Check sheet for the modelled part. Datum: model origin and axes. Units: mm. Coordinates: 2 decimals unless noted, no trailing zeros. Order: outer loops, then holes, each group sorted by start corner. A loop starts at its lowest first (then second) coordinate and runs counter-clockwise, first axis right, second up.
from build123d import *

# Parameters (mm, degrees)
SM_BASE_FLANGE_1_DEPTH      = 746
HOLE_WIZARD_M41_D           = 3.3
HOLE_WIZARD_M41_DEPTH       = 11.5
HOLE_WIZARD_M41_CSINK_D     = 4.05
HOLE_WIZARD_M41_CSINK_ANGLE = 90
HOLE_WIZARD_M41_TIP         = 0.991420021
HOLE_WIZARD_M61_D           = 6.6
HOLE_WIZARD_M61_DEPTH       = 59
HOLE_WIZARD_M61_TIP         = 1.982840043


# Sheet-metal steps are written as plain solids
with BuildPart() as part:
    # Sketch 1 → Базовая кромка1 (new body)
    with BuildSketch(Plane.XY):
        with BuildLine():
            Line((0, 40), (0, 3.8))
            ThreePointArc((0, 3.8), (1.112994231, 1.112994231), (3.8, 0))
            Line((3.8, 0), (30, 0))
            Line((30, 0), (30, 2))
            Line((30, 2), (3.8, 2))
            ThreePointArc((3.8, 2), (2.527207794, 2.527207794), (2, 3.8))
            Line((2, 3.8), (2, 40))
            Line((2, 40), (0, 40))
        make_face()
    extrude(amount=SM_BASE_FLANGE_1_DEPTH)

    # Отверстие обработанное метчиком M41
    with Locations(Plane(origin=(0, 0, 0), x_dir=(-1, 0, 0), z_dir=(0, -1, 0))):
        with Locations((-15, -18), (-15, -89), (-15, -160), (-15, -231), (-15, -302), (-15, -373), (-15, -444), (-15, -515), (-15, -586), (-15, -657), (-15, -728)):
            CounterSinkHole(HOLE_WIZARD_M41_D / 2, HOLE_WIZARD_M41_CSINK_D / 2, depth=HOLE_WIZARD_M41_DEPTH, counter_sink_angle=HOLE_WIZARD_M41_CSINK_ANGLE)
            with Locations((0, 0, -(HOLE_WIZARD_M41_DEPTH + HOLE_WIZARD_M41_TIP / 2))):  # 118° drill point
                Cone(0, HOLE_WIZARD_M41_D / 2, HOLE_WIZARD_M41_TIP, mode=Mode.SUBTRACT)

    # Отверстие с зазором M61
    with Locations(Plane.ZY):
        with Locations((561, 25), (545, 25), (185, 25), (201, 25)):
            Hole(HOLE_WIZARD_M61_D / 2, depth=HOLE_WIZARD_M61_DEPTH)
            with Locations((0, 0, -(HOLE_WIZARD_M61_DEPTH + HOLE_WIZARD_M61_TIP / 2))):  # 118° drill point
                Cone(0, HOLE_WIZARD_M61_D / 2, HOLE_WIZARD_M61_TIP, mode=Mode.SUBTRACT)


solid = part.part
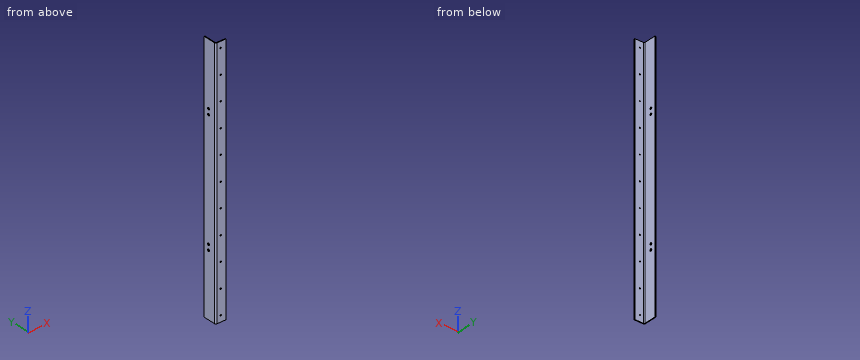
(1) Cross-section at B-B (y = 10). Enter the section's corners in (x, z).
Filled in:
outline: (0, 0) - (2, 0) - (2, 746) - (0, 746) - close
(2) Cross-section at A-A (z = 423). Enter the section's corners in (x, y).
Filled in:
outline: (0, 3.8) arc R3.8 ccw to (3.8, 0) - (30, 0) - (30, 2) - (3.8, 2) arc R1.8 cw to (2, 3.8) - (2, 40) - (0, 40) - close
(3) Thickness scan on probe 1 along Y at (x, z) = (23.5, 570.5); probe 2 along X at (y, z) = (1.35, 89). Record the ranges inside material, lowest first.
Filled in:
probe 1: y = 0 to 2
probe 2: x = 0.9 to 13.35, 16.65 to 30
(4) Go/stop test with flat-tipped pins: P1, Ø4.5, axis at x = 15, z = 586, coming from the +Y side; P2, Ø3, axis at x = 15, z = 231, coming from the +Y side; P3, Ø18, axis at y = 22, z = 254.5, coming from the +X side; P4, Ø4, axis at x = 15, z = 373, coming from the -Y side (3 decimals). Record where each tip stops, or that it passes through.
Filled in:
P1: stops at y = 2
P2: passes through
P3: stops at x = 2
P4: stops at y = 0.025
